Can you work these out from the model? Positions are in its coordinate system, mm. A direction names the side the tool comes from. Give positions to 0.01 mm unless a question says otherwise; leave off trailing zeros. Order: outer loops, then holes, each group sorted by start corner. A loop starts at its lowest first (then second) coordinate and runs counter-clockwise, first axis right, second up. Notation, with made-up numbers: (-28, 15.25) - (8, 15.25) arc R23 cw to (8, 39.25) - close; hole circle Ø4 at (15.5, 87.25). An arc over 180 degrees is marked (long way). Answer as CSV lines item,"result".
```python
from build123d import *

# Parameters (mm, degrees)
BOSS_EXTRUDE1_DEPTH      = 20
BOSS_EXTRUDE1_DEPTH_BACK = 5
BOSS_EXTRUDE2_DEPTH      = 5
BOSS_EXTRUDE3_DEPTH      = 271


with BuildPart() as part:
    # Sketch1 → Boss-Extrude1 (new body, two sides)
    with BuildSketch(Plane.XY) as boss_extrude1_sk:
        with BuildLine():
            Line((0, 25), (0, 17))
            ThreePointArc((0, 17), (-17, 0), (0, -17))
            Line((0, -17), (0, -25))
            ThreePointArc((0, -25), (-25, 0), (0, 25))
        make_face()
    extrude(amount=BOSS_EXTRUDE1_DEPTH)
    extrude(boss_extrude1_sk.sketch, amount=-BOSS_EXTRUDE1_DEPTH_BACK)

    # Sketch2 → Boss-Extrude2 (add)
    with BuildSketch(Plane.XY):
        with BuildLine():
            Line((0, 25), (0, 77))
            Line((0, 77), (-65, 77))
            Line((-65, 77), (-65, 32.113081447))
            ThreePointArc((-65, 32.113081447), (-61.581037686, -38.262590053), (0, -72.5))
            Line((0, -72.5), (0, -25))
            ThreePointArc((0, -25), (-25, 0), (0, 25))
        make_face()
    extrude(amount=-BOSS_EXTRUDE2_DEPTH)


with BuildPart() as body_2:
    # Mirror2: mirrored copy
    add(part.part.mirror(Plane.XY.offset(-140.5)))


with BuildPart() as part_1:
    add(part.part)

    add(body_2.part)  # Boss-Extrude3 merges body 2
    # Sketch3 → Boss-Extrude3 (add)
    with BuildSketch(Plane(origin=(0, 0, -5), x_dir=(-1, 0, 0), z_dir=(0, 0, -1))):
        with BuildLine():
            Line((60, 77), (60, 30.923292192))
            ThreePointArc((60, 30.923292192), (57.634938288, -35.134938288), (0, -67.5))
            Line((0, -67.5), (0, -72.5))
            ThreePointArc((0, -72.5), (61.581037686, -38.262590053), (65, 32.113081447))
            Line((65, 32.113081447), (65, 77))
            Line((65, 77), (60, 77))
        make_face()
    extrude(amount=BOSS_EXTRUDE3_DEPTH)


solid = part_1.part
```
1) Which directions (+Z, -Z, +X, -X, +Y, -Y) give clear straight access to the entire face, cutting with the end or side of a thin tool? Please do faces 4 (the flat face through (-60, 54, -139)), 5 (the flat face through (-65, 54, -139)), 6 (the cylindrical face through (-24.994, -0.55, -291.14)), 7 (the cylindrical face through (-24.994, -0.55, 10.14)).
Answer block:
face 4,"+X, +Y"
face 5,"+Z, -Z, -X, +Y"
face 6,"-Z, -X"
face 7,"+Z, -X"
2) I want a section at A-A on z = -172.5. Write out the boundary of the cut face in (x, y), plus the area to 3 significant figures.
Answer block:
outline,"(-65, 32.11) arc R72.5 ccw to (0, -72.5) - (0, -67.5) arc R67.5 cw to (-60, 30.92) - (-60, 77) - (-65, 77) - close"
area,"941 mm2"
3) If we mould it in two halves opening along Y, with no side actions, what happens to faces 1 (the cylindrical face through (-58.13, -34.31, -138.6)), 2 (the flat face through (0, -69, -140)), 3 (the flat face through (-62, 77, -98))? For each: +Y half, -Y half, draft (parallel to the pull), parting line (faces both ways), or undercut.
Answer block:
face 1,"undercut"
face 2,"draft"
face 3,"+Y half"
4) I need wall thicknesses on line 1 along Z through (x, y) = (-15, -21.5); line 2 along X through (y, z) = (-2, -14.5); line 3 along X through (y, z) = (48, -225). Which ranges of each line are inside material? Lowest first, please. Write a range as [from, to].
Answer block:
line 1,"[-281, -276], [-5, 0]"
line 2,"[-72.47, -67.47]"
line 3,"[-65, -60]"
5) I want a section at C-C on x = -36. Write out the boundary of the cut face in (y, z).
Answer block:
outline,"(-62.93, -281) - (77, -281) - (77, -276) - (-57.1, -276) - (-57.1, -5) - (77, -5) - (77, 0) - (-62.93, 0) - close"
6) I'm going to push flat-ended pins straight in: P1, Ø6, axis at x = -42, y = 60, coming from the +Z side; P2, Ø22.5, axis at y = 45.5, z = -121, coming from the -X side; P3, Ø3, axis at y = -12.5, z = -225, coming from the +X side. Where does each tip first touch, or does it pass through?
Answer block:
P1,"z = 0"
P2,"x = -65"
P3,"x = -66.03"
7) I want a section at B-B on y = 0. Write out the boundary of the cut face in (x, z).
Answer block:
outline,"(-72.5, -281) - (-25, -281) - (-25, -301) - (-17, -301) - (-17, -276) - (-67.5, -276) - (-67.5, -5) - (-17, -5) - (-17, 20) - (-25, 20) - (-25, 0) - (-72.5, 0) - close"
